Autodesk Inventor part; units mm, degrees
ref_plane "YZ Plane" through (0, 0, 0) normal (1, 0, 0) x (0, 1, 0)
ref_plane "XZ Plane" through (0, 0, 0) normal (0, 1, 0) x (-1, 0, 0)
ref_plane "XY Plane" through (0, 0, 0) normal (0, 0, 1) x (1, 0, 0)
sketch "Boceto1" plane through (0, 0, 0) normal (0, 1, 0) x (-1, 0, 0)
  line L0 (0, 0) -> (80, 0)
  line L1 (80, 0) -> (80, -80)
  line L2 (80, -80) -> (0, -80)
  line L3 (0, -80) -> (0, 0)
  dimension "d0" = 80
  dimension "d1" = 80
extrude "Extrusión1" add sketch "Boceto1" along normal blind 7
sketch "Boceto2" plane through (0, 0, 0) normal (0, -1, 0) x (1, 0, 0)
  point P0 (0, 0)
sketch "Boceto3" plane through (0, 0, 0) normal (0, -1, 0) x (1, 0, 0)
  line L0 (-80, 0) -> (0, 0) construction
  line L1 (-40, 0) -> (-40, -80) construction
  line L2 (0, -80) -> (-80, -80) construction
  line L3 (-80, -80) -> (-80, 0) construction
  line L4 (-80, -40) -> (0, -40) construction
  line L5 (0, 0) -> (0, -80) construction
  circle A0 centre (-40, -40) radius 27.5
  dimension "d4" = 55
extrude "Extrusión2" add sketch "Boceto3" along normal blind 24
hole "Agujero1" at (-40, 0, -40) direction (0, 1, 0) diameter 40 end through all both
sketch "Boceto4" plane through (0, 7, 0) normal (0, 1, 0) x (1, 0, 0)
  circle A0 centre (-40, 40) radius 20
  line L0 (-40, 40) -> (-40, 80)
  line L1 (0, 80) -> (-80, 80)
  line L2 (0, 80) -> (0, 40)
  line L3 (0, 0) -> (0, 80)
  line L4 (-40, 40) -> (0, 40)
  point P0 (-20, 40)
  point P1 (-40, 60)
extrude "Extrusión3" cut sketch "Boceto4" against normal through all contours A0 L0 L1 L2 L4
sketch "Boceto7" plane through (0, 7, 0) normal (0, 1, 0) x (1, 0, 0)
  line L0 (-40, 40) -> (-57.5963, 22.4037) construction
  line L1 (-80, 40) -> (0, 40) construction
  line L2 (-58.6139, 17.8506) -> (-50.0833, 26.3811)
  line L3 (-50.0833, 26.3811) -> (-53.6189, 29.9167)
  line L4 (-53.6189, 29.9167) -> (-62.1494, 21.3861)
  line L5 (-62.1494, 21.3861) -> (-58.6139, 17.8506)
  point P0 (0, 0)
  point P1 (-60.3816, 19.6184)
  dimension "d16" = 135
  dimension "d17" = 2.5
  dimension "d18" = 2.5
  dimension "d19" = 12.064
sketch3d "Boceto 3D1"
properties part number "Parctica final.xx"
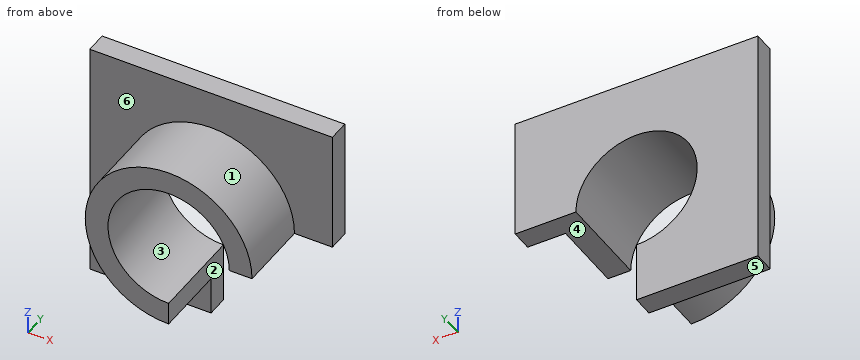
Source: CAD feature listing. Evaluate the final solid. Frame: model axes, mm. Face numbers are marked on the shaded views. A direction names the side the tool comes from. Round coordinates to 2 decimals unless told otherwise and drop trailing zeros. Loops run counter-clockwise (first coordinate to the right, second up) from the corner with the lowest first, then second, coordinate; pieces in that order, holes last. Notation, with made-up numbers: (-35.75, -19.75) -> (7.25, -19.75) arc R11 cw to (7.25, -14.75) -> close; hole circle Ø4 at (14.5, 52.25). An arc over 180 degrees is marked (long way). Answer as a JSON object with one key per item and string values. Group by question number.
Q1. Contact query for flat-ended pins moving along their axis: P1, Ø10, axis at x = -10, y = -2.5, coming from the +Z side; P2, Ø5, axis at y = -19, z = -35, coming from the +X side; P3, Ø5, axis at y = -19, z = -63.5, coming from the +X side; P4, Ø1, axis at x = -19, y = -19, coming from the -Z side. Output: stop coordinate, or through.
Q2. Section query C-C (x = -7). Output: boundary loops of the cut face in (y, z), plus the area to 3 significant figures.
Q3. Section query B-B (z = -28). Output: boundary loops of the cut face in (x, y), plus the area to 3 significant figures.
Q4. Mould query, pull axis X, two halves, no side actions, for the marked faces 1, 2, 3 and 4. Classes: pulls with the +X half, pulls with the -X half, needs draft (parallel to the pull), parting line crosses it, or undercut.
Q5. Ray query, line 1 (Y direction, x = -45.5, z = -10.5); line 2 (X direction, y = -18, z = -32.5); line 3 (X direction, y = -1, z = -37). Return the intervals inside material, ascending. Write a range as from..to.
Q6. Access query for the marked faces 5 and 6. Directions: +Z, -Z, +X, -X, +Y, -Y. A direction counts if a zero-diameter tool reaches every point of the face in a straight line with its end or side. Return the directions, or none.
Q7. Section query D-D (y = -10.5). Output: boundary loops of the cut face in (x, z).
Q8. Section query A-A (x = -48). Output: boundary loops of the cut face in (y, z).
Completed:
{
 "1": {"P1": "z = 0", "P2": "x = -12.61", "P3": "x = -40", "P4": "z = -40"},
 "2": {"outline": "(0, -40) -> (7, -40) -> (7, 0) -> (0, 0) -> close", "area": "280 mm²"},
 "3": {"outline": "(-80, 0) -> (-64.74, 0) -> (-64.74, -24) -> (-56, -24) -> (-56, 7) -> (-80, 7) -> close; (-24, -24) -> (-15.26, -24) -> (-15.26, 0) -> (0, 0) -> (0, 7) -> (-24, 7) -> close", "area": "756 mm²"},
 "4": {"face 1": "parting line crosses it", "face 2": "pulls with the +X half", "face 3": "undercut", "face 4": "needs draft"},
 "5": {"line 1": "0..7", "line 2": "-66.46..-58.54, -21.46..-13.54", "line 3": "-67.34..-59.77, -20.23..-12.66"},
 "6": {"face 5": "-Z, +X, -X, +Y, -Y", "face 6": "-Y"},
 "7": {"outline": "(-40, -67.5) -> (-40, -60) arc R20 cw (long way) to (-20, -40) -> (-12.5, -40) arc R27.5 ccw (long way) to start"},
 "8": {"outline": "(-24, -66.31) -> (0, -66.31) -> (0, -80) -> (7, -80) -> (7, -58.33) -> (-24, -58.33) -> close; (-24, -21.67) -> (7, -21.67) -> (7, 0) -> (0, 0) -> (0, -13.69) -> (-24, -13.69) -> close"}
}
